from build123d import *

# Parameters (mm, degrees)
SKETCH1_R                        = 1
ESP_BRACKET_DEPTH                = 3
SKETCH2_R                        = 1
LORA_HOLDER_SIDES_DEPTH          = 4
SKETCH9_W                        = 21
SKETCH9_H                        = 27
LORA_BACKING_ADD_MPU_HOLE_DEPTH  = 0.5
SKETCH4_W                        = 8
SKETCH4_H                        = 29
LORA_CONNECTOR_COVER_DEPTH       = 2
SKETCH6_W                        = 10.5
SKETCH6_H                        = 29
OTHER_SIDE_LORA_COVER_DEPTH      = 1
LORA_CLAMP_THIRD_SCREWHOLE_REACH = 54.569
SKETCH7_R                        = 1
SKETCH10_R                       = 1
BAROMETER_MOUNT_DEPTH            = 3
ALL_TABS_EXTRUDE_SIDEWAYS_REACH  = 54.872
SKETCH11_W                       = 5.5
SKETCH11_H                       = 1.5
SCREWHOLE_CUT_DEPTH              = 56.118055118
SCREWHOLE_CUT_DEPTH_BACK         = 56.118055118
SKETCH14_R                       = 1
SCREWHOLE_TAB_FILLETS_R          = 2


with BuildPart() as part:
    # Sketch1 → ESP Bracket (new body)
    with BuildSketch(Plane.XY):
        with BuildLine():
            Line((-13, 44), (-13, 0))
            ThreePointArc((-13, 0), (-12.267766953, -1.767766953), (-10.5, -2.5))
            Line((-10.5, -2.5), (10.5, -2.5))
            ThreePointArc((10.5, -2.5), (12.267766953, -1.767766953), (13, 0))
            Line((13, 0), (13, 44))
            ThreePointArc((13, 44), (12.267766953, 45.767766953), (10.5, 46.5))
            Line((10.5, 46.5), (-10.5, 46.5))
            ThreePointArc((-10.5, 46.5), (-12.267766953, 45.767766953), (-13, 44))
        make_face()
        with Locations((-10.5, 44)):
            Circle(SKETCH1_R, mode=Mode.SUBTRACT)
        with Locations((10.5, 44)):
            Circle(SKETCH1_R, mode=Mode.SUBTRACT)
        with Locations((10.5, 0)):
            Circle(SKETCH1_R, mode=Mode.SUBTRACT)
        with Locations((-10.5, 0)):
            Circle(SKETCH1_R, mode=Mode.SUBTRACT)
        with BuildLine():
            Line((-10.5, 41.5), (-10.5, 2.5))
            ThreePointArc((-10.5, 2.5), (-8.732233047, 1.767766953), (-8, 0))
            Line((-8, 0), (8, 0))
            ThreePointArc((8, 0), (8.732233047, 1.767766953), (10.5, 2.5))
            Line((10.5, 2.5), (10.5, 41.5))
            Line((10.5, 41.5), (-10.5, 41.5))
        make_face(mode=Mode.SUBTRACT)
    extrude(amount=-ESP_BRACKET_DEPTH)

    # Sketch2 → LoRa Holder Sides (add)
    with BuildSketch(Plane(origin=(0, 0, -3), x_dir=(-1, 0, 0), z_dir=(0, 0, -1))):
        with BuildLine():
            Line((-8.050510257, 43.5), (8.050510257, 43.5))
            ThreePointArc((8.050510257, 43.5), (10.5, 46.5), (12.949489743, 43.5))
            Line((12.949489743, 43.5), (23.5, 43.5))
            Line((23.5, 43.5), (23.5, 26.5))
            Line((23.5, 26.5), (21.5, 26.5))
            Line((21.5, 26.5), (21.5, 41.5))
            Line((21.5, 41.5), (-21.5, 41.5))
            Line((-21.5, 41.5), (-21.5, 16.5))
            Line((-21.5, 16.5), (21.5, 16.5))
            Line((21.5, 16.5), (21.5, 18))
            Line((21.5, 18), (23.5, 18))
            Line((23.5, 18), (23.5, 16.5))
            Line((23.5, 16.5), (23.5, 14.5))
            Line((23.5, 14.5), (-23.5, 14.5))
            Line((-23.5, 14.5), (-23.5, 43.5))
            Line((-23.5, 43.5), (-12.949489743, 43.5))
            ThreePointArc((-12.949489743, 43.5), (-10.5, 46.5), (-8.050510257, 43.5))
        make_face()
        with Locations(Location((-10.5, 44, 0), (0, 0, 180))):
            Circle(SKETCH2_R, mode=Mode.SUBTRACT)
        with Locations(Location((10.5, 44, 0), (0, 0, 180))):
            Circle(SKETCH2_R, mode=Mode.SUBTRACT)
    extrude(amount=LORA_HOLDER_SIDES_DEPTH)

    # Sketch9 → LoRa Backing (ADD MPU HOLE) (add)
    with BuildSketch(Plane.XY.offset(-3)):
        with Locations((0, 28)):
            Rectangle(SKETCH9_W, SKETCH9_H)
    extrude(amount=LORA_BACKING_ADD_MPU_HOLE_DEPTH)

    # Sketch4 → LoRa Connector Cover (add)
    with BuildSketch(Plane(origin=(0, 0, -7), x_dir=(-1, 0, 0), z_dir=(0, 0, -1))):
        with Locations((-19.5, 29)):
            Rectangle(SKETCH4_W, SKETCH4_H)
    extrude(amount=LORA_CONNECTOR_COVER_DEPTH)

    # Sketch6 → Other Side LoRa Cover (add)
    with BuildSketch(Plane.XY.offset(-3)):
        with Locations((-18.25, 29)):
            Rectangle(SKETCH6_W, SKETCH6_H)
        Polygon((13, 16.5), (13, 14.5), (23.5, 14.5), (23.5, 43.5), (13, 43.5), (13, 41.5), (21.5, 41.5), (21.5, 16.5), align=None)
    extrude(amount=OTHER_SIDE_LORA_COVER_DEPTH)

    # LoRa Clamp Third Screwhole: up to this face of the body (flat: up to its plane)
    lora_clamp_third_screwhole_end = Plane(part.part.faces().sort_by_distance((-18.25, 29, -2))[0])
    # Sketch7 → LoRa Clamp Third Screwhole (add, up to the picked face)
    with BuildSketch(Plane(origin=(0, 0, -7), x_dir=(-1, 0, 0), z_dir=(0, 0, -1)), mode=Mode.PRIVATE) as lora_clamp_third_screwhole_sk1:
        with BuildLine():
            Line((16.5, 16.5), (11.5, 16.5))
            Line((11.5, 16.5), (11.5, 13.5))
            ThreePointArc((11.5, 13.5), (14, 11), (16.5, 13.5))
            Line((16.5, 13.5), (16.5, 16.5))
        make_face()
        with Locations((14, 13.5)):
            Circle(SKETCH7_R, mode=Mode.SUBTRACT)
    lora_clamp_third_screwhole_tool1 = split(extrude(lora_clamp_third_screwhole_sk1.sketch, amount=-LORA_CLAMP_THIRD_SCREWHOLE_REACH, mode=Mode.PRIVATE), bisect_by=lora_clamp_third_screwhole_end, keep=Keep.BOTH, mode=Mode.PRIVATE)
    add(lora_clamp_third_screwhole_tool1.solids().sort_by(Axis((-14, 16.42567, -7), (0, 0, 1)))[0])

    # Sketch10 → Barometer Mount (add)
    with BuildSketch(Plane.XY):
        with BuildLine():
            Line((-10.5, 16.5), (10.5, 16.5))
            Line((10.5, 16.5), (10.5, 14.5))
            Line((10.5, 14.5), (7.5, 14.5))
            Line((7.5, 14.5), (7.5, 12))
            ThreePointArc((7.5, 12), (5, 9.5), (2.5, 12))
            Line((2.5, 12), (2.5, 14.5))
            Line((2.5, 14.5), (-2.5, 14.5))
            Line((-2.5, 14.5), (-2.5, 12))
            ThreePointArc((-2.5, 12), (-5, 9.5), (-7.5, 12))
            Line((-7.5, 12), (-7.5, 14.5))
            Line((-7.5, 14.5), (-10.5, 14.5))
            Line((-10.5, 14.5), (-10.5, 16.5))
        make_face()
        with Locations((-5, 12)):
            Circle(SKETCH10_R, mode=Mode.SUBTRACT)
        with Locations((5, 12)):
            Circle(SKETCH10_R, mode=Mode.SUBTRACT)
    extrude(amount=-BAROMETER_MOUNT_DEPTH)

    # All tabs extrude sideways: up to this face of the body (flat: up to its plane)
    all_tabs_extrude_sideways_end = Plane(part.part.faces().sort_by_distance((-18.166447268, 28.59721894, -2))[0])
    # Sketch11 → All tabs extrude sideways (add, up to the picked face)
    with BuildSketch(Plane(origin=(0, 0, -9), x_dir=(-1, 0, 0), z_dir=(0, 0, -1)), mode=Mode.PRIVATE) as all_tabs_extrude_sideways_sk1:
        with Locations((-26.25, 42.75)):
            Rectangle(SKETCH11_W, SKETCH11_H)
    all_tabs_extrude_sideways_tool1 = split(extrude(all_tabs_extrude_sideways_sk1.sketch, amount=-ALL_TABS_EXTRUDE_SIDEWAYS_REACH, mode=Mode.PRIVATE), bisect_by=all_tabs_extrude_sideways_end, keep=Keep.BOTH, mode=Mode.PRIVATE)
    # Sketch11 → All tabs extrude sideways (add, up to the picked face)
    with BuildSketch(Plane(origin=(0, 0, -9), x_dir=(-1, 0, 0), z_dir=(0, 0, -1)), mode=Mode.PRIVATE) as all_tabs_extrude_sideways_sk2:
        with Locations((-26.25, 15.25)):
            Rectangle(SKETCH11_W, SKETCH11_H)
    all_tabs_extrude_sideways_tool2 = split(extrude(all_tabs_extrude_sideways_sk2.sketch, amount=-ALL_TABS_EXTRUDE_SIDEWAYS_REACH, mode=Mode.PRIVATE), bisect_by=all_tabs_extrude_sideways_end, keep=Keep.BOTH, mode=Mode.PRIVATE)
    # Sketch11 → All tabs extrude sideways (add, up to the picked face)
    with BuildSketch(Plane(origin=(0, 0, -9), x_dir=(-1, 0, 0), z_dir=(0, 0, -1)), mode=Mode.PRIVATE) as all_tabs_extrude_sideways_sk3:
        with Locations((26.25, 15.25)):
            Rectangle(SKETCH11_W, SKETCH11_H)
    all_tabs_extrude_sideways_tool3 = split(extrude(all_tabs_extrude_sideways_sk3.sketch, amount=-ALL_TABS_EXTRUDE_SIDEWAYS_REACH, mode=Mode.PRIVATE), bisect_by=all_tabs_extrude_sideways_end, keep=Keep.BOTH, mode=Mode.PRIVATE)
    # Sketch11 → All tabs extrude sideways (add, up to the picked face)
    with BuildSketch(Plane(origin=(0, 0, -9), x_dir=(-1, 0, 0), z_dir=(0, 0, -1)), mode=Mode.PRIVATE) as all_tabs_extrude_sideways_sk4:
        with Locations((26.25, 42.75)):
            Rectangle(SKETCH11_W, SKETCH11_H)
    all_tabs_extrude_sideways_tool4 = split(extrude(all_tabs_extrude_sideways_sk4.sketch, amount=-ALL_TABS_EXTRUDE_SIDEWAYS_REACH, mode=Mode.PRIVATE), bisect_by=all_tabs_extrude_sideways_end, keep=Keep.BOTH, mode=Mode.PRIVATE)
    add(all_tabs_extrude_sideways_tool1.solids().sort_by(Axis((26.25, 42.75, -9), (0, 0, 1)))[0])
    add(all_tabs_extrude_sideways_tool2.solids().sort_by(Axis((26.25, 15.25, -9), (0, 0, 1)))[0])
    add(all_tabs_extrude_sideways_tool3.solids().sort_by(Axis((-26.25, 15.25, -9), (0, 0, 1)))[0])
    add(all_tabs_extrude_sideways_tool4.solids().sort_by(Axis((-26.25, 42.75, -9), (0, 0, 1)))[0])

    # Sketch14 → Screwhole cut (cut, two sides: drawn at the far end of the back side and taken through both)
    with BuildSketch(Plane(origin=(0, 43.5, 0), x_dir=(1, 0, 0), z_dir=(0, 1, 0)).offset(-SCREWHOLE_CUT_DEPTH_BACK)):
        with Locations(Location((-26.5, 5.5, 0), (0, 0, 90))):
            Circle(SKETCH14_R)
        with Locations(Location((26.5, 5.5, 0), (0, 0, 270))):
            Circle(SKETCH14_R)
    extrude(amount=SCREWHOLE_CUT_DEPTH + SCREWHOLE_CUT_DEPTH_BACK, mode=Mode.SUBTRACT)

    # Screwhole tab fillets
    screwhole_tab_fillets_edges = [part.edges().sort_by_distance(p)[0] for p in [
        (29, 42.75, -9),
        (29, 42.75, -2),
        (29, 15.25, -9),
        (29, 15.25, -2),
        (-29, 15.25, -9),
        (-29, 15.25, -2),
        (-29, 42.75, -9),
        (-29, 42.75, -2),
    ]]
    fillet(screwhole_tab_fillets_edges, radius=SCREWHOLE_TAB_FILLETS_R)


solid = part.part
Here's how the part is built. I have some questions about the finished solid (model axes, mm). A direction names the side the tool comes from. Give positions to 0.01 mm unless a question says otherwise; leave off trailing zeros. Order: outer loops, then holes, each group sorted by start corner. A loop starts at its lowest first (then second) coordinate and runs counter-clockwise, first axis right, second up. Notation, with made-up numbers: M 84.5,36.25 L 106.5,36.25 A26 cw 106.5,75.25 Z; hole C -25,66 d1. An arc over 180 degrees is marked long. Answer as a JSON object with one key per item and string values. Group by question number.
1) On a 3-axis mill with a long thin cutter (end or side, diameter ignored), from which of +Z, -Z, +X, -X, +Y, -Y can I reach the whole of each face in a straight line? I mean faces 3 (the flat face through (-21.5, 34, -5)), 4 (the flat face through (10.5, 8, -1)), 5 (the flat face through (23.5, 29, -5)), 6 (the flat face through (-4.96, 13.15, -3)), 7 (the flat face through (-4, 15, -7)). Say none if no direction works.
2) Suppose I cut it at A-A, the plane x = -5. Write out the boundary of the cut face in (y, z), plus the area to 3 significant figures.
3) Suppose I cut it at D-D, the plane z = -1. Count the separate pieces of the cut face and the enclosed holes in it, plus the area to 3 significant figures.
4) I'm going to push flat-ended pins straight in: pin 1 Ø0.6 at (y, z) = (33, -8) entering from -X; pin 2 Ø3 at (y, z) = (35, -2) entering from +X; pin 3 Ø1.5 at (x, z) = (-9.5, -4) entering from +Y; pin 4 Ø1.2 at (x, y) = (-10.5, 44) entering from +Z. Where does each tip first touch, or does it pass through?
5) Suppose I cut it at C-C, the plane y = 22.5. Write out the boundary of the cut face in (x, z), plus the area to 3 significant figures.
6) Suppose I cut it at B-B, the plane x = -14. Write out the boundary of the cut face in (y, z), plus the area to 3 significant figures.
7) Please list where these lines run through material, in increasing order: L1, parallel to X at y = 15.5, z = -5.5; L2, parallel to Y at x = 5, z = -1.7; L3, parallel to Y at x = -14, z = -5.5. Write a range as [from, to].
8) We'd pull the mould along Y, two halves only. Please class faces 1 (the flat face through (0.9, -0.3, -3)), 2 (the flat face through (25.68, 16, -6.33)): pulls with the +Y half, pulls with the -Y half, needs draft (parallel to the pull), parting line crosses it, or undercut.
Results found:
{
 "1": {"face 3": "-Z", "face 4": "+Z, -Z", "face 5": "+Z, -Z, +X", "face 6": "-Z, +X, -Y", "face 7": "-Z, +Y, -Y"},
 "2": {"outline": "M -2.5,-3 L 0,-3 L 0,0 L -2.5,0 Z; M 9.5,-3 L 11,-3 L 11,0 L 9.5,0 Z; M 13,-3 L 14.5,-3 L 14.5,-7 L 16.5,-7 L 16.5,-3 L 41.5,-3 L 41.5,-7 L 43.5,-7 L 43.5,-3 L 46.5,-3 L 46.5,0 L 41.5,0 L 41.5,-2.5 L 16.5,-2.5 L 16.5,0 L 13,0 Z", "area": "66.0 mm²"},
 "3": {"separate pieces": "1", "enclosed holes": "8", "area": "475 mm²"},
 "4": {"pin 1": "x = 15.5", "pin 2": "x = 23.5", "pin 3": "y = 46.49", "pin 4": "through"},
 "5": {"outline": "M -23.5,-3 L 13,-3 L 13,0 L 10.5,0 L 10.5,-2.5 L -10.5,-2.5 L -10.5,0 L -13,0 L -13,-2 L -23.5,-2 Z; M 15.5,-9 L 23.5,-9 L 23.5,-2 L 21.5,-2 L 21.5,-7 L 15.5,-7 Z", "area": "62.0 mm²"},
 "6": {"outline": "M 11,-7 L 12.5,-7 L 12.5,-2 L 11,-2 Z; M 14.5,-7 L 16.5,-7 L 16.5,-3 L 41.5,-3 L 41.5,-7 L 43.5,-7 L 43.5,-2 L 14.5,-2 Z", "area": "52.5 mm²"},
 "7": {"L1": "[-29, -27.5], [-25.5, 25.5], [27.5, 29]", "L2": "[-2.5, 0], [9.5, 11], [13, 16.5], [41.5, 46.5]", "L3": "[11, 12.5], [14.5, 16.5], [41.5, 43.5]"},
 "8": {"face 1": "needs draft", "face 2": "undercut"}
}
